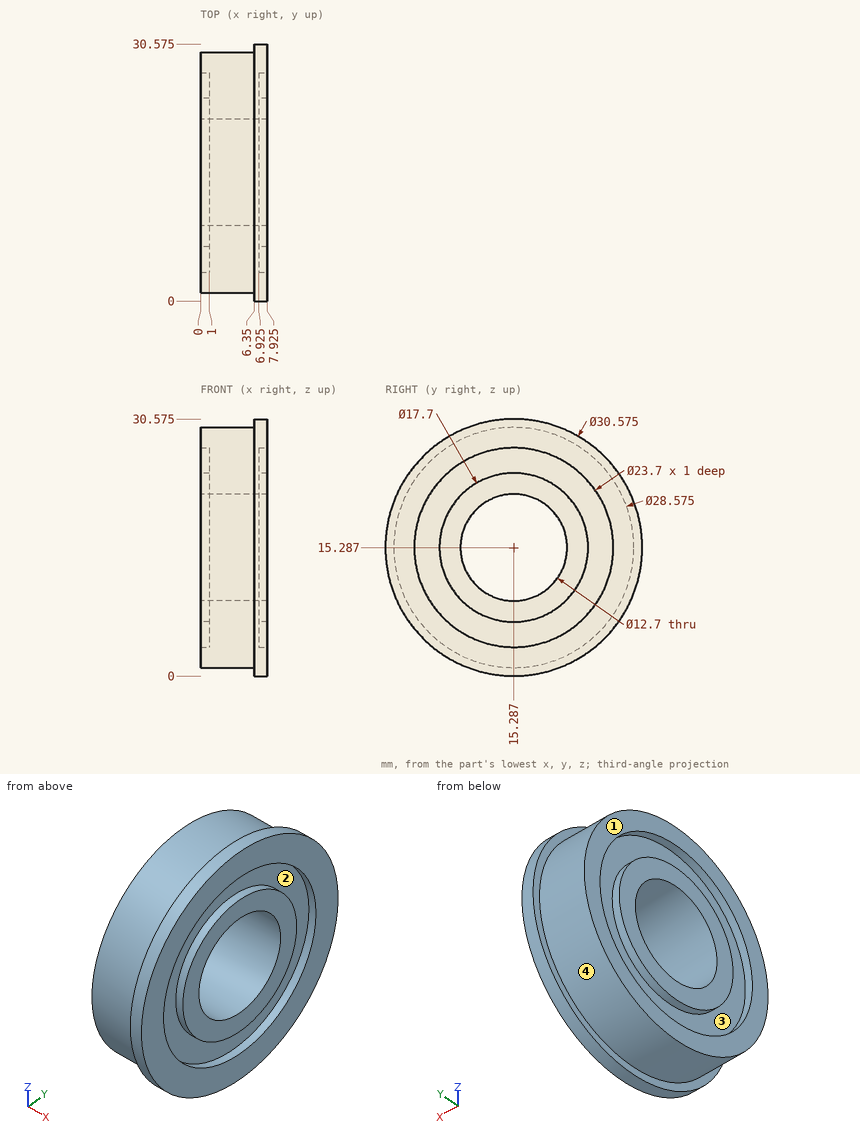
Here's the drawing with two shaded views (mm, measured from the low corner). I have some questions. Give positions to 0.01 mm unless a question says otherwise; leave off trailing zeros. Use one line per item in the form item = value. Start each with the question number.
(1) Please list where these lines run through material, in increasing order: line 1 (Y direction, x = 2, z = 15) (1 decimal); line 2 (X direction, y = 21, z = 24) (1 decimal); line 3 (Y direction, x = 3.75, z = 16).
(2) I'm going to push flat-ended pins straight in: P1, Ø1, axis at x = 6, y = 26, coming from the -Z side; P2, Ø1, axis at x = 1.5, y = 23.5, coming from the -Z side; P3, Ø1, axis at x = 7, z = 16.5, coming from the -Y side; P4, Ø6, axis at y = 23.5, z = 3.5, coming from the -X side. Where does each tip first touch, or does it pass through?
(3) Thinking about a two-plate mould opening in Y: for the marked faces 1, 2, 3 and 4, which applies, released by +Y, released by -Y, zero draft, split by the parting line, or undercut?
Worked out:
q1.line_1 = 1 to 8.9, 21.6 to 29.6
q1.line_2 = 1 to 6.9
q1.line_3 = 1.02 to 8.98, 21.6 to 29.56
q2.P1 = 4.04
q2.P2 = 3.26
q2.P3 = 0.02
q2.P4 = 0
q3.face_1 = zero draft
q3.face_2 = undercut
q3.face_3 = undercut
q3.face_4 = split by the parting line
